Here's how the part is built. I have some questions about the finished solid (model axes, mm). Face numbers are marked on the shaded views. Give positions to 0.01 mm unless a question says otherwise; leave off trailing zeros. Write each loop counter-clockwise with the first axis right and the second up, starting at its lowest first coordinate (ties: lowest second). Pieces come first, ordered by that corner, then holes. Notation, with made-up numbers: (-27.75, 45) -> (-7.75, 45) arc R21 ccw to (-7.75, 81) -> close; hole circle Ø3 at (84, 49.5). An arc over 180 degrees is marked (long way). Return JSON: item names as keys, results as strings.
from build123d import *

# Parameters (mm, degrees)
SKETCH_R        = 70
SKETCH_R_2      = 2.5
PAD_DEPTH       = 10
CHAMFER_SIZE    = 1
CHAMFER001_SIZE = 0.5


with BuildPart() as part:
    # Sketch → Pad (new body)
    with BuildSketch(Plane.XY):
        with BuildLine():
            ThreePointArc((72.327497, 4.998325), (-72.5, 0.00084), (72.327381, -5))
            Line((78, -5), (72.327381, -5))
            ThreePointArc((78, -5), (83, 0), (78, 5))
            Line((72.327497, 4.998325), (78, 5))
        make_face()
        Circle(SKETCH_R, mode=Mode.SUBTRACT)
        with Locations((78, 0)):
            Circle(SKETCH_R_2, mode=Mode.SUBTRACT)
    extrude(amount=PAD_DEPTH)

    # Chamfer
    chamfer_edges = [part.edges().sort_by_distance(p)[0] for p in [
        (-70, 0, 10),
    ]]
    chamfer(chamfer_edges, length=CHAMFER_SIZE)

    # Chamfer001
    chamfer001_edges = [part.edges().sort_by_distance(p)[0] for p in [
        (75.5, 0, 10),
    ]]
    chamfer(chamfer001_edges, length=CHAMFER001_SIZE)


solid = part.part
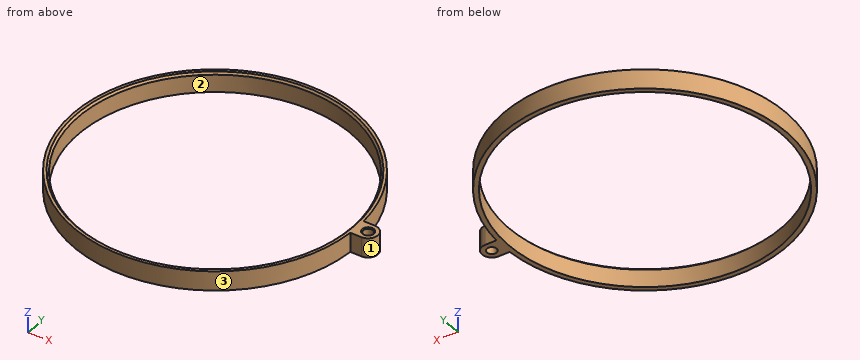
1. If I drill on line 1 (Y direction, x = 0, z = 2); line 2 (Y direction, x = 78, z = 6.5); line 3 (X direction, y = -6, z = 7.5), over which ranges is the centre line in solid material (lowest first)? Write a range as [from, to].
Taken from the geometry:
{"line 1": "y = [-72.5, -70], [70, 72.5]", "line 2": "y = [-5, -2.5], [2.5, 5]", "line 3": "x = [-72.25, -69.74], [69.74, 72.25]"}
2. Suppose I cut it at C-C, the plane z = 7.5. List the corners of the cut face in (x, y) for me, and give its area (3 significant figures).
Taken from the geometry:
{"outline": "(72.33, -5) -> (78, -5) arc R5 ccw to (78, 5) -> (72.33, 5) arc R72.5 ccw (long way) to start; hole circle Ø140 at (0, 0); hole circle Ø5 at (78, 0)", "area": "1,190 mm²"}
3. Suppose I cut it at A-A, the plane x = 0. List the corners of the cut face in (y, z) for me, and give its area (3 significant figures).
Taken from the geometry:
{"outline": "(-72.5, 0) -> (-70, 0) -> (-70, 9) -> (-71, 10) -> (-72.5, 10) -> close; (70, 0) -> (72.5, 0) -> (72.5, 10) -> (71, 10) -> (70, 9) -> close", "area": "49.0 mm²"}
4. If we mould it in two halves opening along X, with no side actions, what happens to the marked faces 1, 2 and 3? For each: released by +X, released by -X, zero draft, split by the parting line, or undercut.
Taken from the geometry:
{"face 1": "released by +X", "face 2": "undercut", "face 3": "split by the parting line"}
5. For pin 1 Ø3 at (y, z) = (15, 7) entering from -X; pin 2 Ø1.7 at (x, z) = (74.5, 4) entering from +Y; pin 3 Ø1.5 at (x, z) = (35.5, 2) entering from -Y, each with a flat end and sliding along its axis, tell me the tip position at first contact or that it passes through.
Taken from the geometry:
{"pin 1": "stops at x = -71.23", "pin 2": "stops at y = 5", "pin 3": "stops at y = -63.63"}
6. Suppose I cut it at B-B, the plane y = 0. List the corners of the cut face in (x, z) for me, and give its area (3 significant figures).
Taken from the geometry:
{"outline": "(-72.5, 0) -> (-70, 0) -> (-70, 9) -> (-71, 10) -> (-72.5, 10) -> close; (70, 0) -> (75.5, 0) -> (75.5, 9.5) -> (75, 10) -> (71, 10) -> (70, 9) -> close; (80.5, 0) -> (83, 0) -> (83, 10) -> (81, 10) -> (80.5, 9.5) -> close", "area": "104 mm²"}
